```python
from build123d import *

# Parameters (mm, degrees)
CROQUIS1_R              = 5
SALIENTE_EXTRUIR1_DEPTH = 33
CROQUIS2_R              = 10
SALIENTE_EXTRUIR2_DEPTH = 2
SKETCH3_R               = 5
SKETCH3_R_2             = 4.5
CUT_EXTRUDE1_DEPTH      = 1


with BuildPart() as part:
    # Croquis1 → Saliente-Extruir1 (new body)
    with BuildSketch(Plane(origin=(0, 0, 0), x_dir=(1, 0, 0), z_dir=(0, 1, 0))):
        Circle(CROQUIS1_R)
    extrude(amount=SALIENTE_EXTRUIR1_DEPTH)

    # Croquis2 → Saliente-Extruir2 (add)
    with BuildSketch(Plane(origin=(0, 33, 0), x_dir=(1, 0, 0), z_dir=(0, 1, 0))):
        Circle(CROQUIS2_R)
    extrude(amount=SALIENTE_EXTRUIR2_DEPTH)

    # Sketch3 → Cut-Extrude1 (cut)
    with BuildSketch(Plane(origin=(0, 2, 0), x_dir=(-1, 0, 0), z_dir=(0, -1, 0))):
        Circle(SKETCH3_R)
        Circle(SKETCH3_R_2, mode=Mode.SUBTRACT)
    extrude(amount=CUT_EXTRUDE1_DEPTH, mode=Mode.SUBTRACT)


solid = part.part
```
The listing builds one solid part. Answer for the finished solid, in the listing's coordinates (mm). A direction names the side the tool comes from. Round coordinates to 2 decimals unless told otherwise and drop trailing zeros. Loops run counter-clockwise (first coordinate to the right, second up) from the corner with the lowest first, then second, coordinate; pieces in that order, holes last.
Q1. Section A-A, the plane x = 0 is taken. Determine the outline of the cut face in (y, z).
Q2. For a pull along Y with two mould halves and no side action, classify faces 1 (the face through (-1.08, 17.28, 4.88)), 2 (the face through (0, 0, 0)), 3 (the face through (0, 35, 0)), 4 (the face through (0.59, 1.51, -4.46)) as released by +Y, released by -Y, zero draft, split by the parting line, or undercut.
Q3. Section D-D, the plane x = 7.5 is taken. Determine the outline of the cut face in (y, z).
Q4. Find the intervals of material crossed by line 1 (Y direction, x = 3, z = 5.25); line 2 (Y direction, x = -0.25, z = -4.75); line 3 (Z direction, x = 0, y = 16.5), in increasing order.
Q5. Section B-B, the plane z = 0 is taken. Determine the outline of the cut face in (x, y), then the cut area to 3 significant figures.
Q6. Section C-C, the plane y = 5 is taken. Determine the outline of the cut face in (x, z), then the cut area to 3 significant figures.
Q7. Which of the six approach directions +Z, -Z, +X, -X, +Y, -Y give full straight-line access (tool end or side, diameter ignored) to faces 5 (the face through (-2.17, 33.99, 9.76)), 6 (the face through (-5, 33, 2))?
Q8. Given pin 1 Ø4 at (x, y) = (2.5, 24.5) entering from -Z; pin 2 Ø10 at (x, y) = (-8, 24) entering from +Z; pin 3 Ø6 at (x, z) = (6, -8) entering from -Y, each flat-ended and moving along its own axis, determine where each tip first touches the part or whether it passes through.
Completed:
1. outline: (0, -5) - (1, -5) - (1, -4.5) - (2, -4.5) - (2, -5) - (33, -5) - (33, -10) - (35, -10) - (35, 10) - (33, 10) - (33, 5) - (2, 5) - (2, 4.5) - (1, 4.5) - (1, 5) - (0, 5) - close
2. face 1: zero draft
2. face 2: released by -Y
2. face 3: released by +Y
2. face 4: undercut
3. outline: (33, -6.61) - (35, -6.61) - (35, 6.61) - (33, 6.61) - close
4. line 1: y = 33 to 35
4. line 2: y = 0 to 1, 2 to 35
4. line 3: z = -5 to 5
5. outline: (-10, 33) - (-5, 33) - (-5, 2) - (-4.5, 2) - (-4.5, 1) - (-5, 1) - (-5, 0) - (5, 0) - (5, 1) - (4.5, 1) - (4.5, 2) - (5, 2) - (5, 33) - (10, 33) - (10, 35) - (-10, 35) - close
5. area: 369 mm2
6. outline: circle Ø10 at (0, 0)
6. area: 78.5 mm2
7. face 5: +Y, -Y
7. face 6: -Y
8. pin 1: stops at z = -4.97
8. pin 2: stops at z = 4
8. pin 3: stops at y = 33
